Autodesk Inventor part; units mm, degrees
ref_plane "Work Plane2" through (50.8025, 3.75, 34.0741) normal (-0.9659, 0, -0.2588) x (0, -1, 0)
ref_plane "YZ Plane" through (0, 0, 0) normal (1, 0, 0) x (0, 1, 0)
ref_plane "XZ Plane" through (0, 0, 0) normal (0, 1, 0) x (-1, 0, 0)
sketch "Sketch1" plane through (0, 0, 0) normal (1, 0, 0) x (0, 1, 0)
  circle A0 centre (0, 0) radius 30.1625
  circle A1 centre (0, 0) radius 34.0741
  dimension "d0" = 60.325
  dimension "d2" = 3.9116
extrude "Extrusion1" add sketch "Sketch1" along normal blind 50.8
sketch "Sketch2" plane through (50.8, 0, 0) normal (1, 0, 0) x (0, 0, -1)
  circle A0 centre (0, 0) radius 30.1625
  circle A1 centre (0, 0) radius 34.0741
  point P0 (-34.0741, 0)
ref_plane "Work Plane1" through (50.8, 0, 34.0741) normal (0, 0, 1) x (1, 0, 0)
sketch "Sketch3" plane through (50.8, 0, 34.0741) normal (0, 0, 1) x (1, 0, 0)
  line L0 (0.0025, 3.75) -> (0.0025, -3.004)
  point P0 (-50.8, 0)
ref_plane "Work Plane2" through (50.8025, 3.75, 34.0741) normal (-0.9659, 0, -0.2588) x (0, -1, 0)
sketch "Sketch4" plane through (50.8025, 3.75, 34.0741) normal (-0.9659, 0, -0.2588) x (0, -1, 0)
  circle A0 centre (3.75, -33.5383) radius 30.1625
  circle A1 centre (3.75, -33.5383) radius 34.0741
  point P0 (3.75, -19.7644)
  dimension "d6" = 60.325
  dimension "d8" = 3.9116
extrude "Extrusion2" add sketch "Sketch4" against normal blind 50.8 and the other way blind 16.51
sketch "Sketch12" plane through (108.5519, 0, 14.8266) normal (0.9659, 0, 0.2588) x (0.2588, 0, -0.9659)
  line L0 (-38.7204, 0) -> (38.3341, 0)
  line L1 (38.3341, 0) -> (38.3341, 2.54)
  line L2 (38.3341, 2.54) -> (-38.7204, 2.54)
  line L3 (-38.7204, 2.54) -> (-38.7204, 0)
  point P0 (-13.7739, 0)
  dimension "d23" = 2.54
extrude "Extrusion5" cut sketch "Sketch12" against normal blind 12.7
sketch "Sketch13" plane through (0, 0, 0) normal (-1, 0, 0) x (0, 0, 1)
  line L0 (-39.4939, 0) -> (40.3288, 0)
  line L1 (40.3288, 0) -> (40.3288, 2.54)
  line L2 (40.3288, 2.54) -> (-39.4939, 2.54)
  line L3 (-39.4939, 2.54) -> (-39.4939, 0)
  dimension "d26" = 2.54
extrude "Extrusion6" cut sketch "Sketch13" against normal blind 12.7
properties part number "pvc_15bend" material "PVC-Piping"
Can you work these out from the model? Positions are in its coordinate system, mm. A direction names the side the tool comes from. Coordinates: 2 decimals unless noted, no trailing zeros. Write each loop counter-clockwise with the first axis right and the second up, starting at its lowest first coordinate (ties: lowest second). Pieces come first, ordered by that corner, then holes. Notation, with made-up numbers: (59, 71) - (83, 71) arc R18 cw to (83, 101) - close; hole circle Ø1 at (28, 37). An arc over 180 degrees is marked (long way). Return JSON: item names as keys, results as strings. Group by question number.
Item 1: Please list where these lines run through material, in increasing order: probe 1 along Z at (x, y) = (15, 0); probe 2 along Y at (x, z) = (74, 9).
Item 2: If we section it at B-B (x = 30): Write out the boundary of the cut face in (y, z) (1 decimal), then the cut area to 3 significant figures.
Item 3: We'd pull the mould along Z, two halves only. Please class faces 1 (the face through (6, 0, 32)), 2 (the face through (50.8, 1.66, 30.38)), 3 (the face through (109.814, 30.06, 10.117)): pulls with the +Z half, pulls with the -Z half, needs draft (parallel to the pull), parting line crosses it, or undercut.
Item 4: I'm going to push flat-ended pins straight in: pin 1 Ø1.3 at (y, z) = (1.5, 31.5) entering from -X; pin 2 Ø5.5 at (x, z) = (109, -17) entering from -Y; pin 3 Ø3 at (x, z) = (5.5, 33) entering from +Y. Where does each tip first touch, or does it pass through?
Item 5: If we section it at A-A (y = 12.5): Write out the boundary of the cut face in (x, z).
Item 6: Which directions (+Z, -Z, +X, -X, +Y, -Y) give clear straight access to the entire face, cutting with the end or side of a thin tool? Please do faces 4 (the face through (87.976, 1.288, 42.538)), 5 (the face through (50.19, -0.39, 30.16)), 6 (the face through (6, 2.54, -32)).
Return value:
{
 "1": {"probe 1": "z = -34.07 to -30.16, 30.16 to 34.07", "probe 2": "y = -33.91 to -29.98, 29.98 to 33.91"},
 "2": {"outline": "circle Ø68.1 at (0, 0); hole circle Ø60.3 at (0, 0)", "area": "789 mm^2"},
 "3": {"face 1": "needs draft", "face 2": "undercut", "face 3": "pulls with the +Z half"},
 "4": {"pin 1": "stops at x = 12.7", "pin 2": "stops at y = -19.26", "pin 3": "stops at y = 12.99"},
 "5": {"outline": "(0, -31.7) - (50.8, -31.7) - (50.8, -29.71) - (51.74, -33.21) - (116.76, -15.79) - (115.66, -11.69) - (50.8, -29.07) - (50.8, -27.45) - (0, -27.45) - close; (0, 27.45) - (35.48, 27.45) - (36.43, 23.92) - (49.6, 27.45) - (50.8, 27.45) - (50.8, 27.77) - (101.45, 41.34) - (100.35, 45.44) - (49.05, 31.7) - (0, 31.7) - close"},
 "6": {"face 4": "+Z, +X", "face 5": "+X", "face 6": "+Z, -Z, -X"}
}
